Could you check a few things on this drawing? It's one solid part, dimensions in mm from its lowest x, y, z. A direction names the side the tool comes from. Round coordinates to 2 decimals unless told otherwise and drop trailing zeros. Write each loop counter-clockwise with the first axis right and the second up, starting at its lowest first coordinate (ties: lowest second). Pieces come first, ordered by that corner, then holes. Notation, with made-up numbers: (57, 13.25) - (93, 13.25) arc R16 cw to (93, 18.25) - close; hole circle Ø1 at (-35.75, 88). An arc over 180 degrees is marked (long way). Use one line per item in the form item = value. Start each with the question number.
1. I want a section at D-D, the plane x = 4.55. List the corners of the cut face in (y, z) for me.
2. I want a section at B-B, the plane x = 3.05. List the corners of the cut face in (y, z) for me.
3. Which directions (+Z, -Z, +X, -X, +Y, -Y) give clear straight access to the entire face, cutting with the end or side of a thin tool? Please do the marked faces 1 and 2.
4. If I drill on line 1 along Z through (x, y) = (4.45, 1.4); line 2 along Z through (x, y) = (2.05, 1.95); line 3 along Y through (x, z) = (2.3, 24), over which ranges is the centre line in solid material (lowest first)?
5. Will these pins go through, and if not, where does the flat tip stop? pin 1 (1 mm diameter, centred on x = 4.5, z = 10.5, fed in from +Y) (1 decimal); pin 2 (2 mm diameter, centred on y = 2.5, z = 16.5, fed in from +X) (3 decimals); pin 3 (0.7 mm diameter, centred on x = 2.5, z = 27.5, fed in from -Y); pin 4 (0.7 mm diameter, centred on x = 2.5, y = 3, fed in from +Z).
6. I want a section at A-A, the plane y = 2.2. List the corners of the cut face in (x, z) for me.
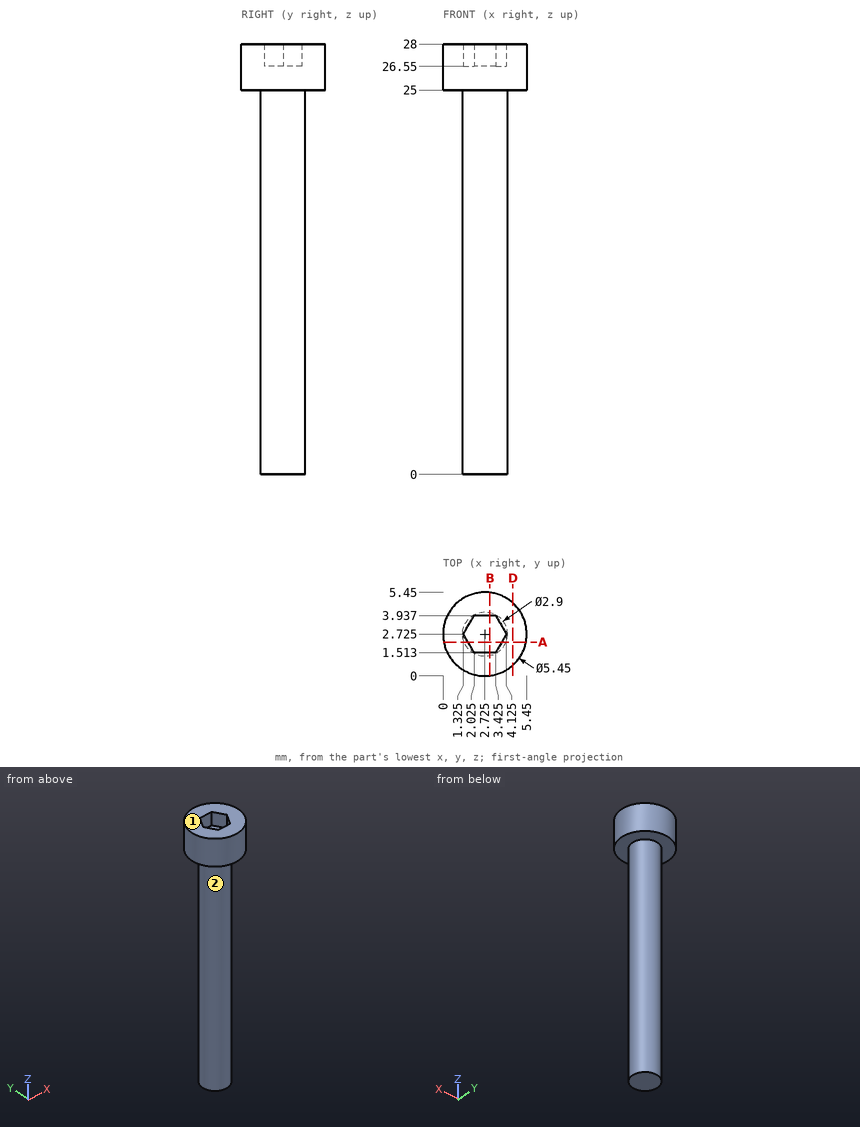
Model answer:
q1.outline = (0.7, 25) - (4.75, 25) - (4.75, 28) - (0.7, 28) - close
q2.outline = (0.02, 25) - (1.31, 25) - (1.31, 0) - (4.14, 0) - (4.14, 25) - (5.43, 25) - (5.43, 28) - (3.94, 28) - (3.94, 26.55) - (1.51, 26.55) - (1.51, 28) - (0.02, 28) - close
q3.face_1 = +Z, +X, -X, +Y, -Y
q3.face_2 = -Z
q4.line_1 = 25 to 28
q4.line_2 = 0 to 26.55
q4.line_3 = 1.34 to 4.11
q5.pin_1 = 3.4
q5.pin_2 = 4.175
q5.pin_3 = 0
q5.pin_4 = 26.55
q6.outline = (0.05, 25) - (1.37, 25) - (1.37, 0) - (4.08, 0) - (4.08, 25) - (5.4, 25) - (5.4, 28) - (3.82, 28) - (3.82, 26.55) - (1.63, 26.55) - (1.63, 28) - (0.05, 28) - close
